Drawing for the job (mm, zero at the part's lowest x, y, z). Coordinates: 2 decimals unless noted, no trailing zeros. Loops run counter-clockwise (first coordinate to the right, second up) from the corner with the lowest first, then second, coordinate; pieces in that order, holes last.
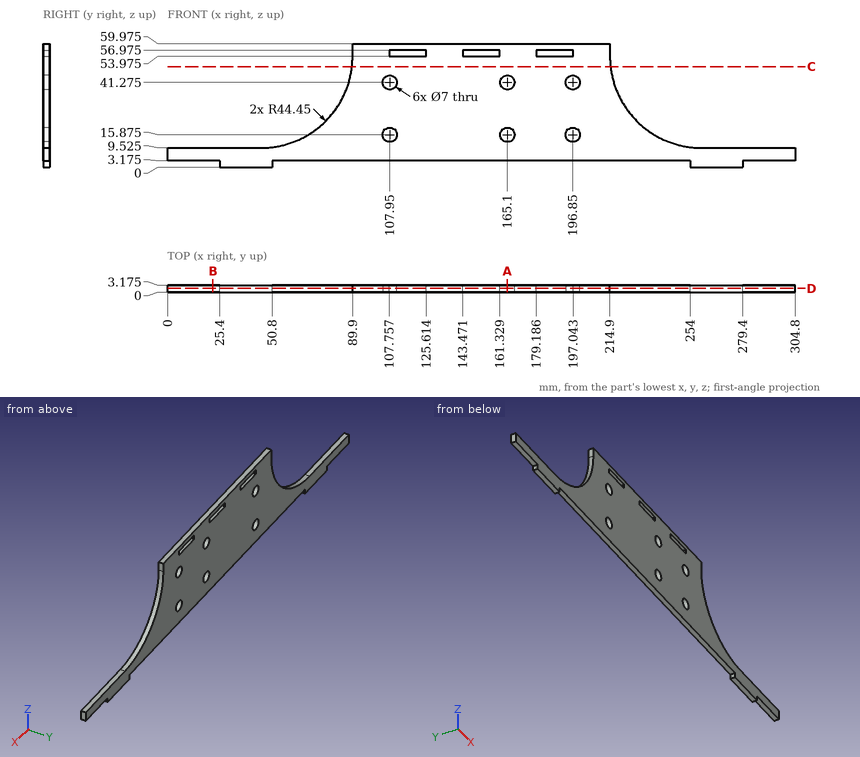
Q1. Drop flat-ended pins along their axis: P1, Ø1, axis at x = 31.5, y = 1, coming from the +Z side (3 decimals); P2, Ø0.9, axis at y = 1.5, z = 55.5, coming from the -X side; P3, Ø1.6, axis at y = 1.5, z = 2, coming from the -X side. Give the stop position or say it passes through.
Q2. Saw through at A-A (x = 165.1). List the corners of the cut face in (y, z) (1 decimal), plus the area to 3 significant figures.
Q3. Probe line 1 (Z direction, x = 196.85, y = 2.1) (1 decimal); line 2 (Z direction, x = 165.1, y = 2.5) (1 decimal); line 3 (X direction, y = 2.55, z = 56.5) (1 decimal). List the from-to ranges inside material, lowest first.
Q4. Saw through at D-D (y = 1.8). Count the separate pieces of the cut face and the enclosed holes in it, plus the area to 3 significant figures.
Q5. Saw through at C-C (z = 49). List the corners of the cut face in (x, y) (1 decimal).
Q6. Saw through at B-B (x = 22). List the corners of the cut face in (y, z) (1 decimal).
Checked values:
1. P1: stops at z = 9.525
1. P2: stops at x = 89.9
1. P3: stops at x = 25.4
2. outline: (0, 3.2) - (3.2, 3.2) - (3.2, 12.4) - (0, 12.4) - close; (0, 19.4) - (3.2, 19.4) - (3.2, 37.8) - (0, 37.8) - close; (0, 44.8) - (3.2, 44.8) - (3.2, 60) - (0, 60) - close
2. area: 136 mm2
3. line 1: z = 3.2 to 12.4, 19.4 to 37.8, 44.8 to 54, 57 to 60
3. line 2: z = 3.2 to 12.4, 19.4 to 37.8, 44.8 to 60
3. line 3: x = 89.9 to 107.8, 125.6 to 143.5, 161.3 to 179.2, 197 to 214.9
4. separate pieces: 1
4. enclosed holes: 9
4. area: 8,860 mm2
5. outline: (89.6, 0) - (215.2, 0) - (215.2, 3.2) - (89.6, 3.2) - close
6. outline: (0, 3.2) - (3.2, 3.2) - (3.2, 9.5) - (0, 9.5) - close
